Could you check a few things on this model? Use its own coordinates, in mm. Face numbers are marked on the shaded views. A direction names the side the tool comes from. Give positions to 0.01 mm unless a question says otherwise; leave off trailing zeros. Loops run counter-clockwise (first coordinate to the right, second up) from the corner with the lowest first, then second, coordinate; pieces in that order, holes last. Notation, with made-up numbers: M -12.5,84.25 L 18.5,84.25 A22 cw 18.5,111.25 Z; hole C 83.25,-26 d9. An arc over 180 degrees is marked long. Use CSV: the item, a comma, the result in double quotes.
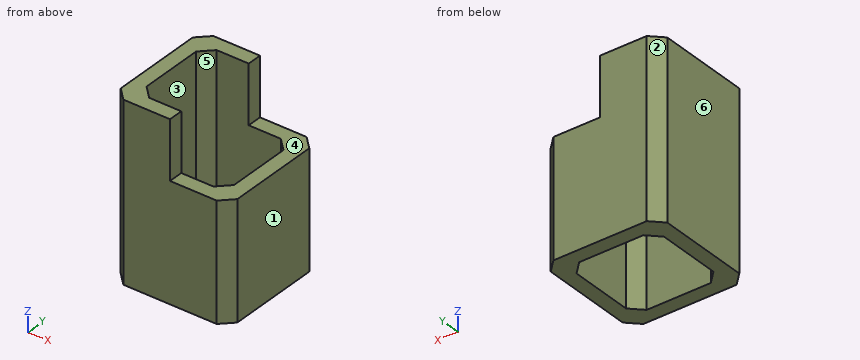
```python
from build123d import *

# Parameters (mm, degrees)
F1_DEPTH = 25.4
F2_W     = 38.1
F2_H     = 38.1
F3_DEPTH = 76.2
F4_SIZE  = 5.08


with BuildPart() as f1:
    # F0 (on Front) → F1 (new body, symmetric)
    with BuildSketch(Plane.XZ):
        Polygon((0, 38.1), (-25.4, 38.1), (-25.4, -38.1), (25.4, -38.1), (25.4, 12.7), (0, 12.7), align=None)
    extrude(amount=F1_DEPTH, both=True)

    # F2 (on face) → F3 (cut, through all)
    with BuildSketch(Plane.XY.offset(38.1)):
        Rectangle(F2_W, F2_H)
    extrude(amount=-F3_DEPTH, mode=Mode.SUBTRACT)

    # F4
    f4_edges = [f1.edges().sort_by_distance(p)[0] for p in [
        (-19.05, -19.05, 0),
        (19.05, -19.05, -12.7),
        (19.05, 19.05, -12.7),
        (-19.05, 19.05, 0),
        (25.4, -25.4, -12.7),
        (25.4, 25.4, -12.7),
        (-25.4, 25.4, 0),
        (-25.4, -25.4, 0),
    ]]
    chamfer(f4_edges, length=F4_SIZE)


solid = f1.part
```
1. If we mould it in two halves opening along Y, with no side actions, what happens to the marked faces 1, 2 and 3? For each: +Y half, -Y half, draft (parallel to the pull), parting line (faces both ways), or undercut.
Outcome:
face 1,"draft"
face 2,"+Y half"
face 3,"undercut"
2. I want a section at A-A, the plane x = 15.5. List the corners of the cut face in (y, z) for me.
Outcome:
outline,"M -25.4,-38.1 L -17.52,-38.1 L -17.52,12.7 L -25.4,12.7 Z; M 17.52,-38.1 L 25.4,-38.1 L 25.4,12.7 L 17.52,12.7 Z"
3. I'm going to push flat-ended pins straight in: pin 1 Ø2 at (x, y) = (17, 6.5) entering from -Z; pin 2 Ø12.5 at (x, y) = (13.5, -0.5) entering from +Z; pin 3 Ø5 at (y, z) = (23.5, 30) entering from +X. Where does each tip first touch, or does it pass through?
Outcome:
pin 1,"through"
pin 2,"z = 12.7"
pin 3,"x = 0"
4. I want a section at C-C, the plane z = 5. List the corners of the cut face in (x, y) for me.
Outcome:
outline,"M -25.4,-20.32 L -20.32,-25.4 L 20.32,-25.4 L 25.4,-20.32 L 25.4,20.32 L 20.32,25.4 L -20.32,25.4 L -25.4,20.32 Z; hole M -19.05,-13.97 L -13.97,-19.05 L 13.97,-19.05 L 19.05,-13.97 L 19.05,13.97 L 13.97,19.05 L -13.97,19.05 L -19.05,13.97 Z"
5. I want a section at D-D, the plane z = 16.5. List the corners of the cut face in (x, y) for me.
Outcome:
outline,"M -25.4,-20.32 L -20.32,-25.4 L 0,-25.4 L 0,-19.05 L -13.97,-19.05 L -19.05,-13.97 L -19.05,13.97 L -13.97,19.05 L 0,19.05 L 0,25.4 L -20.32,25.4 L -25.4,20.32 Z"
6. I want a section at B-B, the plane y = 18. List the corners of the cut face in (x, z) for me.
Outcome:
outline,"M -25.4,-38.1 L -15.02,-38.1 L -15.02,38.1 L -25.4,38.1 Z; M 15.02,-38.1 L 25.4,-38.1 L 25.4,12.7 L 15.02,12.7 Z"
7. Which directions (+Z, -Z, +X, -X, +Y, -Y) give clear straight access to the entire face, cutting with the end or side of a thin tool? Please do the marked faces 4, 5 and 6.
Outcome:
face 4,"+Z, +X, +Y, -Y"
face 5,"+Z, -Z"
face 6,"+Z, -Z, -X, +Y, -Y"
8. Please list where this line runs through material, in increasing order: line 1 (X direction, y = -13, z = -12).
Outcome:
line 1,"-25.4 to -19.05, 19.05 to 25.4"
